Model file for the job. Use its own axes, mm. Face numbers are marked on the shaded views. A direction names the side the tool comes from. Round coordinates to 2 decimals unless told otherwise and drop trailing zeros. Loops run counter-clockwise (first coordinate to the right, second up) from the corner with the lowest first, then second, coordinate; pieces in that order, holes last.
from build123d import *

# Parameters (mm, degrees)
F1_DEPTH = 3
F2_R     = 1.5
F3_R     = 1


with BuildPart() as f1:
    # F0 (on Front) → F1 (new body)
    with BuildSketch(Plane.XZ):
        with BuildLine():
            Line((8.050567, 0.675), (8.050567, -0.675))
            Line((8.050567, -0.675), (4.5, -0.675))
            Line((4.5, -0.675), (4.5, -2.375))
            Line((4.5, -2.375), (9.650567, -2.375))
            Line((9.650567, -2.375), (9.650567, 2.375))
            Line((9.650567, 2.375), (6.905382, 2.375))
            Line((6.905382, 2.375), (6.905382, 10.575))
            Line((6.905382, 10.575), (4.905382, 10.575))
            Line((4.905382, 10.575), (2.005382, 10.575))
            ThreePointArc((2.005382, 10.575), (-0.006672, 6.173255), (-4.5, 4.375))
            Line((-4.5, 4.375), (-6.5, 4.375))
            Line((-6.5, 4.375), (-6.5, 2.375))
            Line((-6.5, 2.375), (-9.650567, 2.375))
            Line((-9.650567, 2.375), (-9.650567, -2.375))
            Line((-9.650567, -2.375), (-4.5, -2.375))
            Line((-4.5, -2.375), (-4.5, -0.675))
            Line((-4.5, -0.675), (-8.050567, -0.675))
            Line((-8.050567, -0.675), (-8.050567, 0.675))
            Line((-8.050567, 0.675), (-4.5, 0.675))
            Line((-4.5, 0.675), (-4.5, 2.375))
            ThreePointArc((-4.5, 2.375), (0.800943, 4.086595), (4.1, 8.575))
            Line((4.1, 8.575), (5, 8.575))
            ThreePointArc((5, 8.575), (4.874797, 5.464936), (4.5, 2.375))
            Line((4.5, 2.375), (4.5, 0.675))
            Line((4.5, 0.675), (8.050567, 0.675))
        make_face()
    extrude(amount=F1_DEPTH)

    # F2
    f2_edges = [f1.edges().sort_by_distance(p)[0] for p in [
        (-6.5, -1.5, 2.375),
        (6.905382, -1.5, 2.375),
        (6.905382, -1.5, 10.575),
        (2.005382, -1.5, 10.575),
    ]]
    fillet(f2_edges, radius=F2_R)

    # F3
    f3_edges = [f1.edges().sort_by_distance(p)[0] for p in [
        (-6.5, -1.5, 4.375),
    ]]
    fillet(f3_edges, radius=F3_R)


solid = f1.part
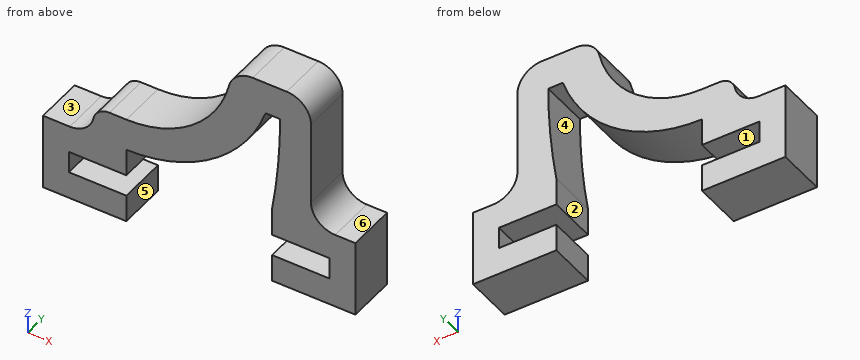
Q1. Flat gauge pins, fed straight in: P1, Ø6, axis at x = 4.5, z = 2, coming from the +Y side; P2, Ø1.2, axis at x = -5, y = -2, coming from the +Z side; P3, Ø0.8, axis at x = -8.5, y = -2, coming from the +Z side (3 decimals); P4, Ø1.5, axis at y = -2, z = 7, coming from the +X side. Where does each tip first touch, or does it go through?
Q2. Tool access for the marked faces 4, 5 and 6: list every direction of +Z, -Z, +X, -X, +Y, -Y with a clear straight run to the whole face (end or side of a thin tool).
Q3. Slice it at C-C on x = 4.75. Give the cut face in (y, z) (3 decimals).
Q4. Probe line 1 (Z direction, x = -5.5, y = -0.2) (3 decimals); line 2 (X direction, y = -1.9, z = 1); line 3 (X direction, y = -2.35, z = 7.25). List the from-to ranges inside material, lowest first.
Q5. Slice it at B-B on x = 7.5. Give the cut face in (y, z) (3 decimals).
Q6. Slice it at A-A on z = -1. Give the cut face in (x, y), plus the area to 3 significant figures.
Q7. Slice it at D-D on x = -3. Give the cut face in (y, z), plus the area to 3 significant figures.
Q8. Pull direction Z, two halves, no side cores. Call the marked faces 1, 2 and 3: pulls with the +Z half, pulls with the -Z half, needs draft (parallel to the pull), parting line crosses it, or undercut.
Reply:
1. P1: stops at y = 0
1. P2: stops at z = 4.38
1. P3: stops at z = 2.375
1. P4: stops at x = 6.91
2. face 4: +Y, -Y
2. face 5: -Z, +Y, -Y
2. face 6: +Z, +X, +Y, -Y
3. outline: (-3, -2.375) - (0, -2.375) - (0, -0.675) - (-3, -0.675) - close; (-3, 0.675) - (0, 0.675) - (0, 4.184) - (-3, 4.184) - close; (-3, 8.575) - (0, 8.575) - (0, 10.575) - (-3, 10.575) - close
4. line 1: z = -2.375 to -0.675, 0.675 to 4.375
4. line 2: x = -9.65 to -4.5, 4.5 to 9.65
4. line 3: x = 0.9 to 3.54, 4.98 to 6.91
5. outline: (-3, -2.375) - (0, -2.375) - (0, -0.675) - (-3, -0.675) - close; (-3, 0.675) - (0, 0.675) - (0, 2.679) - (-3, 2.679) - close
6. outline: (-9.65, -3) - (-4.5, -3) - (-4.5, 0) - (-9.65, 0) - close; (4.5, -3) - (9.65, -3) - (9.65, 0) - (4.5, 0) - close
6. area: 30.9 mm2
7. outline: (-3, 2.5) - (0, 2.5) - (0, 4.55) - (-3, 4.55) - close
7. area: 6.15 mm2
8. face 1: undercut
8. face 2: needs draft
8. face 3: pulls with the +Z half
